from build123d import *

# Parameters (mm, degrees)
BOSS_EXTRUDE1_DEPTH             = 37.19322
BOSS_EXTRUDE2_DEPTH             = 31.75
DRAFT1_ANGLE                    = 12.53
F_1_4_0_25_DIAMETER_HOLE2_D     = 6.35
CUT_EXTRUDE2_DEPTH              = 25.4
F_1_4_0_25_DIAMETER_HOLE3_D     = 6.35
F_1_4_0_25_DIAMETER_HOLE3_DEPTH = 31.75
F_1_4_0_25_DIAMETER_HOLE3_TIP   = 1.907732465
F_1_4_20_TAPPED_HOLE1_D         = 5.1054
F_1_4_20_TAPPED_HOLE1_DEPTH     = 12.7
F_1_4_20_TAPPED_HOLE1_TIP       = 1.533816902


with BuildPart() as part:
    # Sketch1 → Boss-Extrude1 (new body)
    with BuildSketch(Plane(origin=(0, 0, 0), x_dir=(1, 0, 0), z_dir=(0, 1, 0))):
        Polygon((-48.582525221, 30.31081915), (-36.184949557, 27.555802336), (-44.45, -9.636924657), (-56.847575664, -6.881907843), align=None)
    extrude(amount=BOSS_EXTRUDE1_DEPTH)

    # Sketch8 → Boss-Extrude2 (add)
    with BuildSketch(Plane(origin=(0, 0, 0), x_dir=(1, 0, 0), z_dir=(0, 1, 0))):
        Polygon((-36.184949557, 27.555802336), (44.45, 3.063075343), (44.45, -9.636924657), (-44.45, -9.636924657), align=None)
    extrude(amount=BOSS_EXTRUDE2_DEPTH)

    # Draft1
    draft1_faces = [part.faces().sort_by_distance(p)[0] for p in [
        (-52.715050443, 18.59661, -11.714455654),
    ]]
    draft(draft1_faces, Plane.ZX.offset(37.19322), DRAFT1_ANGLE)

    # 1/4 (0.25) Diameter Hole2 (through all)
    with Locations(Plane(origin=(0, 31.75, 0), x_dir=(1, 0, 0), z_dir=(0, 1, 0))):
        with Locations((-6.35, 3.063075343), (19.05, 3.063075343)):
            Hole(F_1_4_0_25_DIAMETER_HOLE2_D / 2)

    # Sketch13 → Cut-Extrude2 (cut)
    with BuildSketch(Plane(origin=(0, 31.75, 0), x_dir=(1, 0, 0), z_dir=(0, 1, 0))):
        with BuildLine():
            Line((-36.184949557, 27.555802336), (-39.910553687, 10.79058375))
            ThreePointArc((-39.910553687, 10.79058375), (-38.665031363, 5.439706394), (-33.711765855, 3.063075343))
            Line((-33.711765855, 3.063075343), (-17.348522628, 3.063075343))
            ThreePointArc((-17.348522628, 3.063075343), (-14.173522628, 3.913814029), (-11.849261314, 6.238075343))
            ThreePointArc((-11.849261314, 6.238075343), (-6.35, 9.413075343), (-0.850738686, 6.238075343))
            ThreePointArc((-0.850738686, 6.238075343), (1.473522628, 3.913814029), (4.648522628, 3.063075343))
            Line((4.648522628, 3.063075343), (8.051477372, 3.063075343))
            ThreePointArc((8.051477372, 3.063075343), (11.226477372, 3.913814029), (13.550738686, 6.238075343))
            ThreePointArc((13.550738686, 6.238075343), (19.05, 9.413075343), (24.549261314, 6.238075343))
            ThreePointArc((24.549261314, 6.238075343), (26.873522628, 3.913814029), (30.048522628, 3.063075343))
            Line((30.048522628, 3.063075343), (44.45, 3.063075343))
            Line((44.45, 3.063075343), (-36.184949557, 27.555802336))
        make_face()
    extrude(amount=-CUT_EXTRUDE2_DEPTH, mode=Mode.SUBTRACT)

    # 1/4 (0.25) Diameter Hole3
    with Locations(Plane.XY.offset(9.636924657)):
        with Locations((38.1, 25.4), (38.1, 12.7), (-25.4, 25.4), (-25.4, 12.7)):
            Hole(F_1_4_0_25_DIAMETER_HOLE3_D / 2, depth=F_1_4_0_25_DIAMETER_HOLE3_DEPTH)
            with Locations((0, 0, -(F_1_4_0_25_DIAMETER_HOLE3_DEPTH + F_1_4_0_25_DIAMETER_HOLE3_TIP / 2))):  # 118° drill point
                Cone(0, F_1_4_0_25_DIAMETER_HOLE3_D / 2, F_1_4_0_25_DIAMETER_HOLE3_TIP, mode=Mode.SUBTRACT)

    # 1/4-20 Tapped Hole1
    with Locations(Plane(origin=(-57.923217538, 13.187114971, -12.87182612), x_dir=(-0.20648022911920935, 0.04700841279958709, 0.977320891063392), z_dir=(-0.9529367695675907, 0.2169507716396215, -0.21176372657057574))):
        with Locations((13.563707416, 17.609083513), (12.340640779, -7.762134727), (-8.941294908, 12.336703083), (-9.552900666, -0.349243556)):
            Hole(F_1_4_20_TAPPED_HOLE1_D / 2, depth=F_1_4_20_TAPPED_HOLE1_DEPTH)
            with Locations((0, 0, -(F_1_4_20_TAPPED_HOLE1_DEPTH + F_1_4_20_TAPPED_HOLE1_TIP / 2))):  # 118° drill point
                Cone(0, F_1_4_20_TAPPED_HOLE1_D / 2, F_1_4_20_TAPPED_HOLE1_TIP, mode=Mode.SUBTRACT)


solid = part.part
Input: part model. Units: mm. Frame: model coordinates. A direction names the side the tool comes from. Coordinates: 2 decimals unless noted, no trailing zeros. Loops run counter-clockwise (first coordinate to the right, second up) from the corner with the lowest first, then second, coordinate; pieces in that order, holes last. Notation, with made-up numbers: (57.5, 35.5) -> (65.5, 35.5) arc R17 cw to (65.5, 44.5) -> close; hole circle Ø3 at (89, 25.5). An arc over 180 degrees is marked (long way). Write each question's results on one line, items separated by ' | '. Start each with the question number.
Q1. Section B-B, the plane x = -26. Return the cut outline in (y, z).
Q2. Pin query (flat end, axial travel): pin 1 (1 mm diameter, centred on x = 6, y = 20.5, fed in from -Z); pin 2 (7.5 mm diameter, centred on x = -25.4, y = 25.4, fed in from +Z); pin 3 (16.5 mm diameter, centred on x = -6.5, z = 4.5, fed in from +Y); pin 4 (3 mm diameter, centred on y = 23.5, z = -1.5, fed in from -X). Return the tip coordinate at first contact, or that it passes through.
Q3. Reachability of faces 1 (the conical face through (-42.84, 9.22, -18.85)), 2 (the cylindrical face through (-38.714, 19.228, -5.502)), 3 (the flat face through (1, 31.75, 2)) from +Z, -Z, +X, -X, +Y, -Y: full face, straight path, thin tool, end or side. Return the list, or none.
Q4. Section D-D, the plane z = -12. Return the cut outline in (x, y).
Q5. Section A-A, the plane x = -6.35. Return the cut outline in (y, z), plus the area to 3 significant figures.
Q6. Pull-direction query (Y, two-part tool) for faces 4 (the conical face through (-40.086, 21.915, -18.239)), 5 (the flat face through (6, 19, -3.063)), 6 (the flat face through (-22, 0, -7)); classes: released by +Y, released by -Y, zero draft, split by the parting line, or undercut.
Q7. Ray query, line 1 (Y direction, x = -25.4, z = 7) (3 decimals); line 2 (X direction, y = 22, z = -0.5); line 3 (X direction, y = 31.5, z = -8). Return the intervals inside material, ascending. Write a range as from..to.
Q8. Section C-C, the plane y = 11. State how many separate pieces and enclosed holes the cut face has, plus the area to 3 significant figures.
Found:
1) outline: (0, -24.46) -> (6.35, -24.46) -> (6.35, -3.06) -> (9.58, -3.06) -> (9.58, 9.64) -> (0, 9.64) -> close; (15.82, -3.06) -> (22.28, -3.06) -> (22.28, 9.64) -> (15.82, 9.64) -> close; (28.52, -3.06) -> (31.75, -3.06) -> (31.75, 9.64) -> (28.52, 9.64) -> close
2) pin 1: z = -3.06 | pin 2: z = 9.64 | pin 3: y = 31.75 | pin 4: x = -58.58
3) face 1: none | face 2: +Y | face 3: +Z, +X, +Y
4) outline: (-61.12, 0) -> (15.03, 0) -> (15.03, 6.35) -> (-39.64, 6.35) -> (-39.64, 37.19) -> (-52.65, 37.19) -> close
5) outline: (0, -18.49) -> (6.35, -18.49) -> (6.35, -9.41) -> (31.75, -9.41) -> (31.75, -6.24) -> (0, -6.24) -> close; (0, 0.11) -> (31.75, 0.11) -> (31.75, 9.64) -> (0, 9.64) -> close | area: 461 mm2
6) face 4: undercut | face 5: zero draft | face 6: released by -Y
7) line 1: 0..9.525, 15.875..22.225, 28.575..31.75 | line 2: -58.67..-8.22, -4.48..17.18, 20.92..44.45 | line 3: -54.84..-39.9, -10.34..-2.36, 15.06..23.04
8) separate pieces: 3 | enclosed holes: 2 | area: 1,710 mm2
